Here's the drawing with two shaded views (mm, measured from the low corner). I have some questions. A direction names the side the tool comes from. Coordinates: 2 decimals unless noted, no trailing zeros. Write each loop counter-clockwise with the first axis right and the second up, starting at its lowest first coordinate (ties: lowest second). Pieces come first, ordered by that corner, then holes.
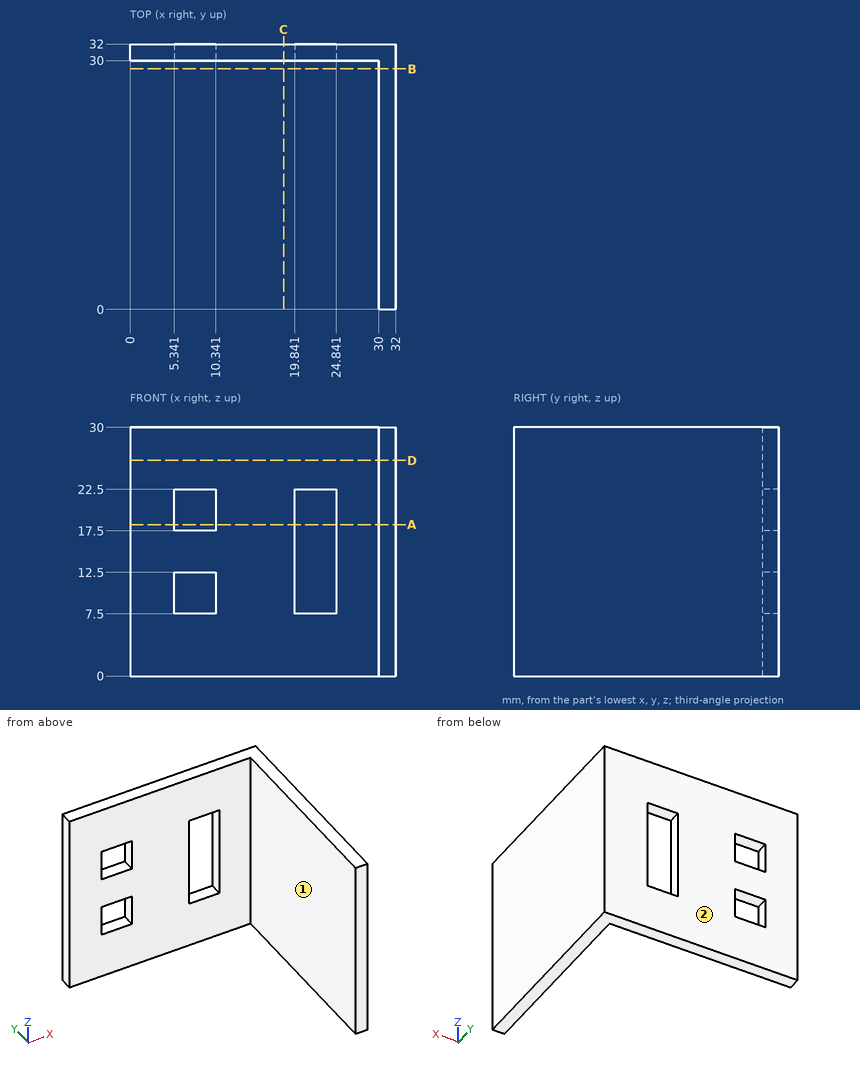
1. On a 3-axis mill with a long thin cutter (end or side, diameter ignored), from which of +Z, -Z, +X, -X, +Y, -Y can I reach the whole of each face in a straight line? I mean the marked faces 1 and 2. Say none if no direction works.
Verdict:
face 1: +Z, -Z, -X, -Y
face 2: +Z, -Z, +X, -X, +Y
2. I want a section at B-B on y = 29. Please give me the cut outline in (x, z).
Verdict:
outline: (30, 0) - (32, 0) - (32, 30) - (30, 30) - close
3. I want a section at A-A on z = 18.25. Please give me the cut outline in (x, y).
Verdict:
outline: (0, 30) - (5.34, 30) - (5.34, 32) - (0, 32) - close; (10.34, 30) - (19.84, 30) - (19.84, 32) - (10.34, 32) - close; (24.84, 30) - (30, 30) - (30, 0) - (32, 0) - (32, 32) - (24.84, 32) - close
4. Please list where this line runs through material, in increasing order: line 1 along Y through (x, z) = (4.5, 14.5).
Verdict:
line 1: y = 30 to 32
5. For pin 1 (8 mm diameter, centred on x = 18, z = 5.5, fed in from -Y); pin 2 (1.5 mm diameter, centred on y = 18.5, z = 13, fed in from -X), each with a flat end and sliding along its axis, tell me the tip position at first contact or that it passes through.
Verdict:
pin 1: stops at y = 30
pin 2: stops at x = 30
6. I want a section at D-D on z = 26. Please give me the cut outline in (x, y).
Verdict:
outline: (0, 30) - (30, 30) - (30, 0) - (32, 0) - (32, 32) - (0, 32) - close
